Study the drawing (mm; zero at the part's minimum x, y, z) and answer. Coordinates: 2 decimals unless noted, no trailing zeros. Order: outer loops, then holes, each group sorted by start corner. A loop starts at its lowest first (then second) coordinate and runs counter-clockwise, first axis right, second up.
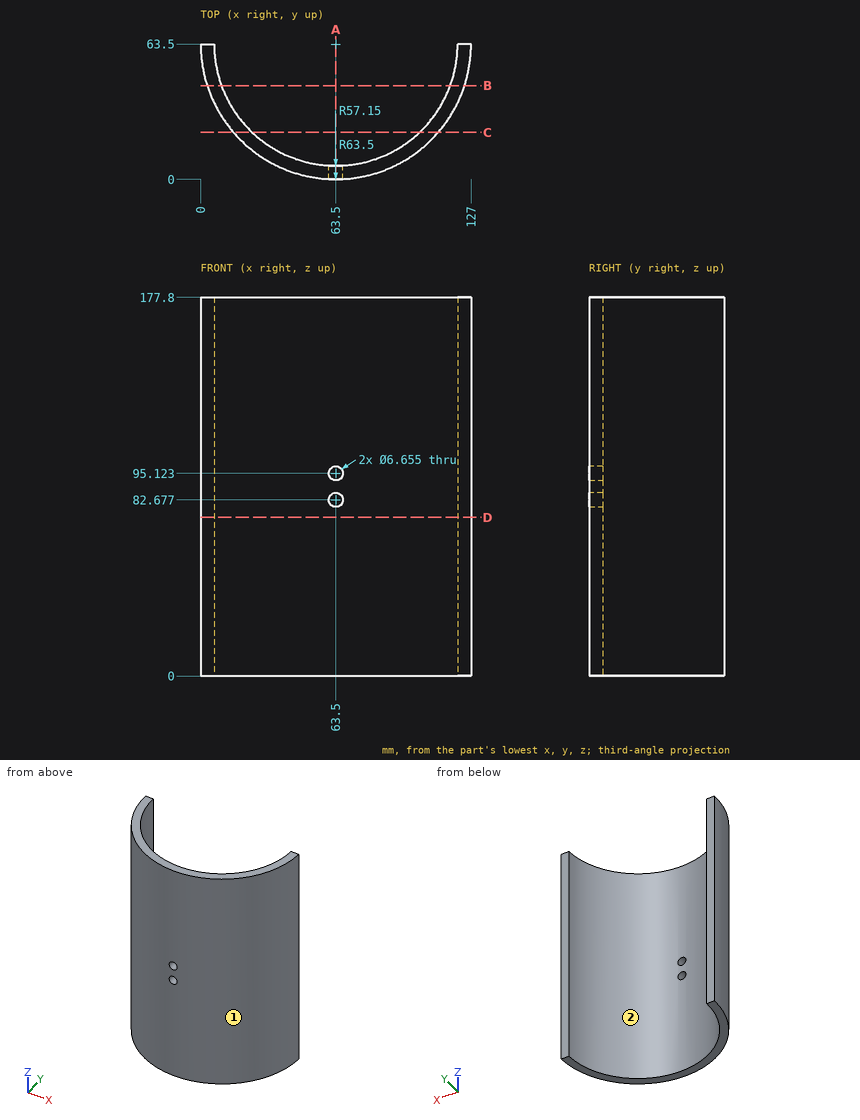
1) A cutting plane is placed at B-B, the plane y = 44. Determine the outline of the cut face in (x, z), and give its area (3 significant figures).
A:
outline: (3.07, 0) - (9.78, 0) - (9.78, 177.8) - (3.07, 177.8) - close; (117.22, 0) - (123.93, 0) - (123.93, 177.8) - (117.22, 177.8) - close
area: 2,390 mm2
2) Flat-ended cylindrical pins translate along their axes: pin 1 Ø1 at (y, z) = (44, 55) entering from +X; pin 2 Ø5 at (x, z) = (72.5, 149.5) entering from -Y; pin 3 Ø3 at (x, z) = (14, 37) entering from +Y; pin 4 Ø4 at (x, z) = (63.5, 82.677) entering from +Y. Find the tip coordinate at first contact, or state that the pin passes through.
A:
pin 1: stops at x = 124.09
pin 2: stops at y = 0.33
pin 3: stops at y = 37.71
pin 4: passes through
3) Straight lines are drawn through the part: line 1 (Z direction, x = 63, y = 5); line 2 (X direction, y = 58.5, z = 59.5); line 3 (X direction, y = 31, z = 33). For each, find the intervals that lie inside material, in ascending order.
A:
line 1: z = 0 to 79.39, 85.97 to 91.83, 98.41 to 177.8
line 2: x = 0.2 to 6.57, 120.43 to 126.8
line 3: x = 8.95 to 16.49, 110.51 to 118.05
4) A cutting plane is placed at D-D, the plane z = 74.5. Determine the outline of the cut face in (x, y), and give its area (3 significant figures).
A:
outline: (0, 63.5) arc R63.5 ccw to (127, 63.5) - (120.65, 63.5) arc R57.15 cw to (6.35, 63.5) - close
area: 1,200 mm2
5) Determine the mould class of the marked faces 1 and 2 for opening direction X: pulls with the +X half, pulls with the -X half, needs draft (parallel to the pull), parting line crosses it, or undercut.
A:
face 1: parting line crosses it
face 2: undercut
6) A cutting plane is placed at C-C, the plane y = 22. Determine the outline of the cut face in (x, z), and give its area (3 significant figures).
A:
outline: (15.44, 0) - (24.21, 0) - (24.21, 177.8) - (15.44, 177.8) - close; (102.79, 0) - (111.56, 0) - (111.56, 177.8) - (102.79, 177.8) - close
area: 3,120 mm2
7) A cutting plane is placed at A-A, the plane x = 63.5. Determine the outline of the cut face in (y, z).
A:
outline: (0, 0) - (6.35, 0) - (6.35, 79.35) - (0, 79.35) - close; (0, 86) - (6.35, 86) - (6.35, 91.8) - (0, 91.8) - close; (0, 98.45) - (6.35, 98.45) - (6.35, 177.8) - (0, 177.8) - close
